from build123d import *
from build123d import SkipClean  # not in build123d's __all__

# Parameters (mm, degrees)
F1_DEPTH    = 3.75
F3_D        = 3.3
F3_DEPTH    = 12.2
F3_TIP      = 0.9914200214
F4_R        = 2
F5_T4_DEPTH = 7.5
F5_S5_R     = 1.65
F5_T6_DEPTH = 7
F6_SIZE     = 0.5
F8_D        = 6.8


# Not quite as in the source:
# - a fillet or chamfer that OpenCascade refuses, or shapes differently, is made with other operations: its cross-section is extruded or revolved along the edge and cut away or added
# - a feature names something its author has since deleted; it is built from what else it names


with BuildPart() as f1:
    # F0 (on Front) → F1 (new body, symmetric)
    with BuildSketch(Plane.XZ):
        with BuildLine():
            ThreePointArc((0, -24), (-24, 0), (0, 24))
            Line((0, 24), (0, 39))
            Line((0, 39), (-7, 39))
            Line((-7, 39), (-7, 28.1424945589))
            ThreePointArc((-7, 28.1424945589), (-22.8473193176, 17.8605710995), (-29, 0))
            ThreePointArc((-29, 0), (-27.9004726433, -13.0232858743), (-31.6552133192, -25.541946259))
            ThreePointArc((-31.6552133192, -25.541946259), (-30.9284075442, -33.5939072683), (-23.3128108861, -36.3077625094))
            ThreePointArc((-23.3128108861, -36.3077625094), (-11.4240360348, -35.6417318474), (0, -39))
            Line((0, -39), (0, -24))
        make_face()
    extrude(amount=F1_DEPTH, both=True)

    # F3
    with Locations(Plane.YZ):
        with Locations((0, 33), (0, -33)):
            Hole(F3_D / 2, depth=F3_DEPTH)
            with Locations((0, 0, -(F3_DEPTH + F3_TIP / 2))):  # 118° drill point
                Cone(0, F3_D / 2, F3_TIP, mode=Mode.SUBTRACT)

    # F4
    f4_edges = [f1.edges().sort_by_distance(p)[0] for p in [
        (-3.5, 3.75, 39),
        (-3.5, -3.75, 39),
        (-11.424036, 3.75, -35.641732),
        (-11.424036, -3.75, -35.641732),
    ]]
    fillet(f4_edges, radius=F4_R)

    # F5: fillet of radius 7 on 1 edges, made by hand


with BuildPart() as f5_tool2:
    # F5_s3 → F5_t4 (new body)
    with BuildSketch(Plane.XZ.offset(-3.75)):
        with BuildLine():
            ThreePointArc((-11.2777777778, 26.7172552556), (-8.1666666667, 29.2968523148), (-7, 33.1662479036))
            Line((-7, 33.1662479036), (-7, 28.1424945589))
            ThreePointArc((-7, 28.1424945589), (-9.1666306182, 27.5131401899), (-11.2777777778, 26.7172552556))
        make_face()
    extrude(amount=F5_T4_DEPTH)

    # F5_s5 → F5_t6 (cut, symmetric)
    with BuildSketch(Plane.YZ.offset(-9.1)):
        with Locations((0, 33)):
            Circle(F5_S5_R)
    with SkipClean():  # cleaning this boolean's faces spoils the solid; the shape is the same uncleaned
        extrude(amount=F5_T6_DEPTH, both=True, mode=Mode.SUBTRACT)


with BuildPart() as f1_1:
    add(f1.part, clean=False)

    # F5_t1: union F5_tool2
    add(f5_tool2.part)

    # F6
    f6_edges = [f1_1.edges().sort_by_distance(p)[0] for p in [
        (-24, 3.75, 0),
        (-24, -3.75, 0),
    ]]
    chamfer(f6_edges, length=F6_SIZE)

    # F8 (through all)
    with Locations(Plane.XZ.offset(3.75)):
        with Locations((-25, -29)):
            Hole(F8_D / 2)


solid = f1_1.part
Geometry check sheet. Reference: the model listing, model coordinates, mm. A direction names the side the tool comes from. Give positions to 0.01 mm unless a question says otherwise; leave off trailing zeros. Answer in a Markdown table with one row per item. Add a question column.
1) Cross-section at A-A on x = -9. State how many separate pieces and enclosed holes the cut face has, and give its area (3 significant figures).
2) Gauge pin test, flat ends, axial feed: P1, Ø2, axis at x = -18, y = 0.5, coming from the +Z side; P2, Ø3, axis at y = -1, z = 15, coming from the +X side; P3, Ø2, axis at y = 0, z = -33, coming from the +X side. Record the tip position at first contact, or that the pin passes through.
3) Material ranges on probe 1 along Z at (x, y) = (-9, 1); probe 2 along Z at (x, y) = (-9, 0); probe 3 along Y at (x, z) = (-2, -33), recorded low to high. Write a range as from..to.
4) Draft check along X on faces 4 (the face through (-3.55, 3.18, 38.4)), 5 (the face through (-24.034, -0.053, 16.228)), 6 (the face through (-28.243, 0.052, -27.979)). Enter one of: pulls with the +X half, pulls with the -X half, needs draft (parallel to the pull), parting line crosses it, or undercut.
5) Set-up check for faces 1 (the face through (-6.185, 0.215, -31.364)), 2 (the face through (-7, 0, 36)), 3 (the face through (-3, 0, 39)): record each of +Z, -Z, +X, -X, +Y, -Y from which the full face is reachable in a straight line by a thin tool's end or side.
Outcome:
| question | item | result |
|---|---|---|
| 1 | separate pieces | 2 |
| 1 | enclosed holes | 1 |
| 1 | area | 137 mm^2 |
| 2 | P1 | stops at z = 23.49 |
| 2 | P2 | stops at x = -17.43 |
| 2 | P3 | stops at x = -12.59 |
| 3 | probe 1 | z = -36.01..-34.31, -31.69..-22.25, 22.25..28.27 |
| 3 | probe 2 | z = -36.01..-34.65, -31.35..-22.25, 22.25..28.27 |
| 3 | probe 3 | y = -3.75..-1.65, 1.65..3.75 |
| 4 | face 4 | needs draft |
| 4 | face 5 | pulls with the -X half |
| 4 | face 6 | undercut |
| 5 | face 1 | +X |
| 5 | face 2 | +Z, -X, +Y, -Y |
| 5 | face 3 | +Z, +X, -X, +Y, -Y |
